```python
from build123d import *

# Parameters (mm, degrees)
SKETCH1_R           = 5
SKETCH1_R_2         = 2.075
SKETCH1_R_3         = 2.05
BOSS_EXTRUDE1_DEPTH = 3.175


with BuildPart() as part:
    # Sketch1 → Boss-Extrude1 (new body)
    with BuildSketch(Plane(origin=(0, 0, 0), x_dir=(-1, 0, 0), z_dir=(0, 0, -1))):
        with BuildLine():
            Line((49, 30), (-49, 30))
            ThreePointArc((-49, 30), (-53.242640687, 28.242640687), (-55, 24))
            Line((-55, 24), (-55, -24))
            ThreePointArc((-55, -24), (-53.242640687, -28.242640687), (-49, -30))
            Line((-49, -30), (49, -30))
            ThreePointArc((49, -30), (53.242640687, -28.242640687), (55, -24))
            Line((55, -24), (55, 24))
            ThreePointArc((55, 24), (53.242640687, 28.242640687), (49, 30))
        make_face()
        with Locations(Location((-30.51, 0, 0), (0, 0, 180))):
            Circle(SKETCH1_R, mode=Mode.SUBTRACT)
        with Locations(Location((30.5, 0, 0), (0, 0, 180))):
            Circle(SKETCH1_R, mode=Mode.SUBTRACT)
        with Locations(Location((-22.51, -8, 0), (0, 0, 180))):
            Circle(SKETCH1_R_2, mode=Mode.SUBTRACT)
        with Locations(Location((-38.51, -8, 0), (0, 0, 180))):
            Circle(SKETCH1_R_2, mode=Mode.SUBTRACT)
        with Locations(Location((-38.51, 8, 0), (0, 0, 180))):
            Circle(SKETCH1_R_2, mode=Mode.SUBTRACT)
        with Locations(Location((-22.51, 8, 0), (0, 0, 180))):
            Circle(SKETCH1_R_2, mode=Mode.SUBTRACT)
        with Locations(Location((38.5, -8, 0), (0, 0, 180))):
            Circle(SKETCH1_R_2, mode=Mode.SUBTRACT)
        with Locations(Location((22.5, -8, 0), (0, 0, 180))):
            Circle(SKETCH1_R_2, mode=Mode.SUBTRACT)
        with Locations(Location((22.5, 8, 0), (0, 0, 180))):
            Circle(SKETCH1_R_2, mode=Mode.SUBTRACT)
        with Locations(Location((38.5, 8, 0), (0, 0, 180))):
            Circle(SKETCH1_R_2, mode=Mode.SUBTRACT)
        with Locations(Location((50, -25, 0), (0, 0, 180))):
            Circle(SKETCH1_R_3, mode=Mode.SUBTRACT)
        with Locations(Location((-50, -25, 0), (0, 0, 180))):
            Circle(SKETCH1_R_3, mode=Mode.SUBTRACT)
        with Locations(Location((-50, 25, 0), (0, 0, 180))):
            Circle(SKETCH1_R_3, mode=Mode.SUBTRACT)
        with Locations(Location((50, 25, 0), (0, 0, 180))):
            Circle(SKETCH1_R_3, mode=Mode.SUBTRACT)
        with BuildLine():
            Line((-42.5, 6.393335184), (-42.5, -6.393335184))
            ThreePointArc((-42.5, -6.393335184), (-42.704196298, -7.945320832), (-43.302886484, -9.391669905))
            Line((-43.302886484, -9.391669905), (-47.200721621, -16.147917476))
            ThreePointArc((-47.200721621, -16.147917476), (-48.887996412, -16.847284721), (-50, -15.398333796))
            Line((-50, -15.398333796), (-50, 15.398333796))
            ThreePointArc((-50, 15.398333796), (-48.887996412, 16.847284721), (-47.200721621, 16.147917476))
            Line((-47.200721621, 16.147917476), (-43.302886484, 9.391669905))
            ThreePointArc((-43.302886484, 9.391669905), (-42.704196298, 7.945320832), (-42.5, 6.393335184))
        make_face(mode=Mode.SUBTRACT)
        with BuildLine():
            Line((-35.034616452, -12), (35.034616452, -12))
            ThreePointArc((35.034616452, -12), (38.035448976, -12.804328324), (40.231729969, -15.001665279))
            Line((40.231729969, -15.001665279), (43.620632646, -20.875763253))
            ThreePointArc((43.620632646, -20.875763253), (43.619971802, -23.625381574), (41.238622284, -25))
            Line((41.238622284, -25), (-41.238622284, -25))
            ThreePointArc((-41.238622284, -25), (-43.619971802, -23.625381574), (-43.620632646, -20.875763253))
            Line((-43.620632646, -20.875763253), (-40.231729969, -15.001665279))
            ThreePointArc((-40.231729969, -15.001665279), (-38.035448976, -12.804328324), (-35.034616452, -12))
        make_face(mode=Mode.SUBTRACT)
        with BuildLine():
            Line((42.5, -6.393335184), (42.5, 6.393335184))
            ThreePointArc((42.5, 6.393335184), (42.704196298, 7.945320832), (43.302886484, 9.391669905))
            Line((43.302886484, 9.391669905), (47.200721621, 16.147917476))
            ThreePointArc((47.200721621, 16.147917476), (48.887996412, 16.847284721), (50, 15.398333796))
            Line((50, 15.398333796), (50, -15.398333796))
            ThreePointArc((50, -15.398333796), (48.887996412, -16.847284721), (47.200721621, -16.147917476))
            Line((47.200721621, -16.147917476), (43.302886484, -9.391669905))
            ThreePointArc((43.302886484, -9.391669905), (42.704196298, -7.945320832), (42.5, -6.393335184))
        make_face(mode=Mode.SUBTRACT)
        with BuildLine():
            Line((35.034616452, 12), (-35.034616452, 12))
            ThreePointArc((-35.034616452, 12), (-38.035448976, 12.804328324), (-40.231729969, 15.001665279))
            Line((-40.231729969, 15.001665279), (-43.620632646, 20.875763253))
            ThreePointArc((-43.620632646, 20.875763253), (-43.619971802, 23.625381574), (-41.238622284, 25))
            Line((-41.238622284, 25), (41.238622284, 25))
            ThreePointArc((41.238622284, 25), (43.619971802, 23.625381574), (43.620632646, 20.875763253))
            Line((43.620632646, 20.875763253), (40.231729969, 15.001665279))
            ThreePointArc((40.231729969, 15.001665279), (38.035448976, 12.804328324), (35.034616452, 12))
        make_face(mode=Mode.SUBTRACT)
    extrude(amount=-BOSS_EXTRUDE1_DEPTH)


solid = part.part
```
Model file for the job. Use its own axes, mm. Give positions to 0.01 mm unless a question says otherwise; leave off trailing zeros. Write each loop counter-clockwise with the first axis right and the second up, starting at its lowest first coordinate (ties: lowest second). Pieces come first, ordered by that corner, then holes. Notation, with made-up numbers: M 27.5,83.5 L 72.5,83.5 A26 ccw 72.5,107.5 Z; hole C 79.25,47 d5. An arc over 180 degrees is marked long. Use a Markdown table: item, result.
1) Cut at C-C (y = -8). List the corners of the cut face in (x, z) (3 decimals), and give its area (3 significant figures).
Responses:
| item | result |
|---|---|
| outline | M -55,0 L -50,0 L -50,3.175 L -55,3.175 Z; M -42.719,0 L -40.575,0 L -40.575,3.175 L -42.719,3.175 Z; M -36.425,0 L -24.575,0 L -24.575,3.175 L -36.425,3.175 Z; M -20.425,0 L 20.435,0 L 20.435,3.175 L -20.425,3.175 Z; M 24.585,0 L 36.435,0 L 36.435,3.175 L 24.585,3.175 Z; M 40.585,0 L 42.719,0 L 42.719,3.175 L 40.585,3.175 Z; M 50,0 L 55,0 L 55,3.175 L 50,3.175 Z |
| area | 250 mm2 |
2) Pull direction X, two halves, no side cores. Call faces 1 (the flat face through (42.5, 0, 2)), 2 (the flat face through (-1, 30, 2)), 3 (the cylindrical face through (-20.58, -7.21, 1.57)), 4 (the flat face through (-55, 0, 2)): +X half, -X half, draft (parallel to the pull), parting line (faces both ways), or undercut.
Responses:
| item | result |
|---|---|
| face 1 | undercut |
| face 2 | draft |
| face 3 | undercut |
| face 4 | -X half |
3) Cut at B-B (x = -12). List the corners of the cut face in (y, z) (3 decimals).
Responses:
| item | result |
|---|---|
| outline | M -30,0 L -25,0 L -25,3.175 L -30,3.175 Z; M -12,0 L 12,0 L 12,3.175 L -12,3.175 Z; M 25,0 L 30,0 L 30,3.175 L 25,3.175 Z |
4) Cut at A-A (y = 0). List the corners of the cut face in (x, z) (3 decimals), and give its area (3 significant figures).
Responses:
| item | result |
|---|---|
| outline | M -55,0 L -50,0 L -50,3.175 L -55,3.175 Z; M -42.5,0 L -35.5,0 L -35.5,3.175 L -42.5,3.175 Z; M -25.5,0 L 25.51,0 L 25.51,3.175 L -25.5,3.175 Z; M 35.51,0 L 42.5,0 L 42.5,3.175 L 35.51,3.175 Z; M 50,0 L 55,0 L 55,3.175 L 50,3.175 Z |
| area | 238 mm2 |
5) Pin check, flat tip, straight feed: pin 1 (2.5 mm diameter, centred on x = 22.51, y = 8, fed in from -Z). Stop position of the tip, or through.
Responses:
| item | result |
|---|---|
| pin 1 | passes through |
6) Cut at D-D (x = -38.5). List the corners of the cut face in (y, z) (3 decimals).
Responses:
| item | result |
|---|---|
| outline | M -30,0 L -25,0 L -25,3.175 L -30,3.175 Z; M -13.102,0 L -10.075,0 L -10.075,3.175 L -13.102,3.175 Z; M -5.925,0 L 5.925,0 L 5.925,3.175 L -5.925,3.175 Z; M 10.075,0 L 13.102,0 L 13.102,3.175 L 10.075,3.175 Z; M 25,0 L 30,0 L 30,3.175 L 25,3.175 Z |
7) Drill centre lines: line 1 (Y direction, x = 22.51, z = 1.25) (3 decimals); line 2 (X direction, y = 5.5, z = 0.95); line 3 (Y direction, x = -25, z = 0.2). Where is each one in solid material? Low to high. Write a range as from..to.
Responses:
| item | result |
|---|---|
| line 1 | y = -30..-25, -12..-10.075, -5.925..5.925, 10.075..12, 25..30 |
| line 2 | x = -55..-50, -42.5..42.5, 50..55 |
| line 3 | y = -30..-25, -12..12, 25..30 |
